from build123d import *

# Parameters (mm, degrees)
RESSALTO_EXTRUS_O1_DEPTH = 25
ESBO_O3_W                = 25
ESBO_O3_H                = 5
RESSALTO_EXTRUS_O2_DEPTH = 20
FILETE1_R                = 10
FILETE2_R                = 10
ESBO_O4_W                = 25
ESBO_O4_H                = 5
RESSALTO_EXTRUS_O3_DEPTH = 20
FILETE3_R                = 10
FILETE4_R                = 10
ESBO_O5_R                = 5
CORTE_EXTRUS_O1_DEPTH    = 20
FILETE5_R                = 2.5
FILETE6_R                = 2.5


with BuildPart() as part:
    # Esboço2 → Ressalto-extrusão1 (new body)
    with BuildSketch(Plane.XY):
        with BuildLine():
            Line((24.097579721, -6.65632418), (29.097579721, -6.65632418))
            Line((29.097579721, -6.65632418), (29.097579721, -36.65632418))
            Line((29.097579721, -36.65632418), (-29.097579721, -36.65632418))
            Line((-29.097579721, -36.65632418), (-29.097579721, -6.65632418))
            Line((-29.097579721, -6.65632418), (-24.097579721, -6.65632418))
            ThreePointArc((-24.097579721, -6.65632418), (0, -25), (24.097579721, -6.65632418))
        make_face()
    extrude(amount=RESSALTO_EXTRUS_O1_DEPTH)

    # Esboço3 → Ressalto-extrusão2 (add)
    with BuildSketch(Plane.ZY.offset(29.097579721)):
        with Locations((12.5, -34.15632418)):
            Rectangle(ESBO_O3_W, ESBO_O3_H)
    extrude(amount=RESSALTO_EXTRUS_O2_DEPTH)

    # Filete1
    filete1_edges = [part.edges().sort_by_distance(p)[0] for p in [
        (-49.097579721, -34.15632418, 25),
    ]]
    fillet(filete1_edges, radius=FILETE1_R)

    # Filete2
    filete2_edges = [part.edges().sort_by_distance(p)[0] for p in [
        (-49.097579721, -34.15632418, 0),
    ]]
    fillet(filete2_edges, radius=FILETE2_R)

    # Esboço4 → Ressalto-extrusão3 (add)
    with BuildSketch(Plane(origin=(29.097579721, 0, 0), x_dir=(0, 0, -1), z_dir=(1, 0, 0))):
        with Locations((-12.5, -34.15632418)):
            Rectangle(ESBO_O4_W, ESBO_O4_H)
    extrude(amount=RESSALTO_EXTRUS_O3_DEPTH)

    # Filete3
    filete3_edges = [part.edges().sort_by_distance(p)[0] for p in [
        (49.097579721, -34.15632418, 25),
    ]]
    fillet(filete3_edges, radius=FILETE3_R)

    # Filete4
    filete4_edges = [part.edges().sort_by_distance(p)[0] for p in [
        (49.097579721, -34.15632418, 0),
    ]]
    fillet(filete4_edges, radius=FILETE4_R)

    # Esboço5 → Corte-extrusão1 (cut)
    with BuildSketch(Plane(origin=(0, -31.65632418, 0), x_dir=(1, 0, 0), z_dir=(0, 1, 0))):
        with Locations((39.097579721, -12.5)):
            Circle(ESBO_O5_R)
        with Locations((-39.097579721, -12.5)):
            Circle(ESBO_O5_R)
    extrude(amount=-CORTE_EXTRUS_O1_DEPTH, mode=Mode.SUBTRACT)

    # Filete5
    filete5_edges = [part.edges().sort_by_distance(p)[0] for p in [
        (-29.097579721, -31.65632418, 12.5),
    ]]
    fillet(filete5_edges, radius=FILETE5_R)

    # Filete6
    filete6_edges = [part.edges().sort_by_distance(p)[0] for p in [
        (29.097579721, -31.65632418, 12.5),
    ]]
    fillet(filete6_edges, radius=FILETE6_R)


solid = part.part
Verification items for the finished model (mm, model axes). A direction names the side the tool comes from. Give positions to 0.01 mm unless a question says otherwise; leave off trailing zeros. Order: outer loops, then holes, each group sorted by start corner. A loop starts at its lowest first (then second) coordinate and runs counter-clockwise, first axis right, second up. Notation, with made-up numbers: M 14.25,-19.5 L 54.25,-19.5 A20 cw 54.25,16.5 Z; hole C 32.25,-21 d1. An arc over 180 degrees is marked long. Use one line per item in the form item = value. Start each with the question number.
Q1. Mould release check, pull along Y, two halves, no side actions. Record for faces 4 (the flat face through (-44, -31.656, 15)), 5 (the flat face through (-1, -36.656, 13)), 6 (the cylindrical face through (-46.09, -34.12, 22.15)): +Y half, -Y half, draft (parallel to the pull), parting line (faces both ways), or undercut.
Q2. Section check A-A (z = 12.5). Enter the section's corners in (x, y), then the cut area to 3 significant figures.
Q3. Section check D-D (z = 5.5). Enter the section's corners in (x, y).
Q4. Go/stop test with flat-tipped pins: pin 1 Ø14 at (x, z) = (37, 6.5) entering from +Y; pin 2 Ø7 at (y, z) = (-15.5, 10.5) entering from -X; pin 3 Ø3 at (x, z) = (-17, 13) entering from +Y. Record where each tip stops, or that it passes through.
Q5. Section check B-B (y = -17.25). Enter the section's corners in (x, z).
Q6. Scan lines: line 1 along X through (y, z) = (-33.15, 12.5); line 2 along X through (y, z) = (-18.75, 13); line 3 along Y through (x, z) = (43, 2.25). Record each from-to range of solid material in increasing order. Write a range as [from, to].
Q7. Access from +Z, -Z, +X, -X, +Y, -Y to the whole of each face (thin tool, end or side, straight path). Record for faces 1 (the cylindrical face through (0, -25, 12)), 2 (the flat face through (29.098, -18, 12)), 3 (the flat face through (-29.098, -18, 12)).
Q8. Section check C-C (x = -42). Enter the section's corners in (y, z), then the cut area to 3 significant figures.
Evaluation:
q1.face_4 = +Y half
q1.face_5 = -Y half
q1.face_6 = draft
q2.outline = M -49.1,-36.66 L -44.1,-36.66 L -44.1,-31.66 L -49.1,-31.66 Z; M -34.1,-36.66 L 34.1,-36.66 L 34.1,-31.66 L 31.6,-31.66 A2.5 cw 29.1,-29.16 L 29.1,-6.66 L 24.1,-6.66 A25 cw -24.1,-6.66 L -29.1,-6.66 L -29.1,-29.16 A2.5 cw -31.6,-31.66 L -34.1,-31.66 Z; M 44.1,-36.66 L 49.1,-36.66 L 49.1,-31.66 L 44.1,-31.66 Z
q2.area = 1,200 mm2
q3.outline = M -48.03,-36.66 L 48.03,-36.66 L 48.03,-31.66 L 31.6,-31.66 A2.5 cw 29.1,-29.16 L 29.1,-6.66 L 24.1,-6.66 A25 cw -24.1,-6.66 L -29.1,-6.66 L -29.1,-29.16 A2.5 cw -31.6,-31.66 L -48.03,-31.66 Z
q4.pin_1 = -31.08
q4.pin_2 = -29.1
q4.pin_3 = -16.82
q5.outline = M -29.1,0 L -18.1,0 L -18.1,25 L -29.1,25 Z; M 18.1,0 L 29.1,0 L 29.1,25 L 18.1,25 Z
q6.line_1 = [-49.1, -44.1], [-34.1, 34.1], [44.1, 49.1]
q6.line_2 = [-29.1, -16.54], [16.54, 29.1]
q6.line_3 = [-36.66, -31.66]
q7.face_1 = +Z, -Z, +Y
q7.face_2 = +Z, -Z, +X, +Y
q7.face_3 = +Z, -Z, -X, +Y
q8.outline = M -36.66,0.43 L -31.66,0.43 L -31.66,8.43 L -36.66,8.43 Z; M -36.66,16.57 L -31.66,16.57 L -31.66,24.57 L -36.66,24.57 Z
q8.area = 80.0 mm2
